Check sheet for the modelled part. Datum: model origin and axes. Units: mm. A direction names the side the tool comes from. Coordinates: 2 decimals unless noted, no trailing zeros. Loops run counter-clockwise (first coordinate to the right, second up) from the corner with the lowest first, then second, coordinate; pieces in that order, holes last. Notation, with made-up numbers: M -0.5,-37.75 L 49.5,-37.75 A19 cw 49.5,-29.75 Z; hole C -23.75,60 d5. An arc over 180 degrees is marked long. Write each question's results on one line, items separated by ' | '. Start each with the question number.
from build123d import *

# Parameters (mm, degrees)
BOSS_EXTRU_2_DEPTH = 2.4
CHANFREIN3_SIZE    = 1.4
CHANFREIN4_SIZE    = 1.4


with BuildPart() as part:
    # Esquisse2 → Boss.-Extru.2 (new body)
    with BuildSketch(Plane(origin=(0, 0, 0), x_dir=(1, 0, 0), z_dir=(0, 1, 0))):
        Polygon((-0.604426001, 3.317657231), (-4.604426001, 3.317657231), (-8.332361087, 1.867657231), (-8.332361087, -0.132342769), (-4.604426001, -1.582342769), (-0.604426001, -1.582342769), (3.123509084, -0.132342769), (3.123509084, 1.867657231), align=None)
        with BuildLine():
            Line((-0.204426001, 1.517657231), (-5.004426001, 1.517657231))
            ThreePointArc((-5.004426001, 1.517657231), (-5.654426001, 0.867657231), (-5.004426001, 0.217657231))
            Line((-5.004426001, 0.217657231), (-0.204426001, 0.217657231))
            ThreePointArc((-0.204426001, 0.217657231), (0.445573999, 0.867657231), (-0.204426001, 1.517657231))
        make_face(mode=Mode.SUBTRACT)
    extrude(amount=BOSS_EXTRU_2_DEPTH)

    # Chanfrein3
    chanfrein3_edges = [part.edges().sort_by_distance(p)[0] for p in [
        (-8.332361087, 2.4, -0.867657231),
    ]]
    chamfer(chanfrein3_edges, length=CHANFREIN3_SIZE)

    # Chanfrein4
    chanfrein4_edges = [part.edges().sort_by_distance(p)[0] for p in [
        (3.123509084, 2.4, -0.867657231),
    ]]
    chamfer(chanfrein4_edges, length=CHANFREIN4_SIZE)


solid = part.part
1) Section check D-D (x = -5.25). Enter the section's corners in (y, z).
2) Release check for a two-part mould opening along X. For faces 1 (the flat face through (-3, 0, 0)), 2 (the cylindrical face through (-5.654, 1.183, -0.882)), 3 (the flat face through (1.29, 1.18, -2.58)) record: +X half, -X half, draft (parallel to the pull), parting line (faces both ways), or undercut.
3) Set-up check for faces 4 (the flat face through (-6.442, 1.183, -2.603)), 5 (the cylindrical face through (0.445, 1.183, -0.853)): record each of +Z, -Z, +X, -X, +Y, -Y from which the full face is reachable in a straight line by a thin tool's end or side.
4) Section check C-C (y = 0.6). Enter the section's corners in (x, z).
5) Section check A-A (x = -3.5). Enter the section's corners in (y, z), then the cut area to 3 significant figures.
6) Thickness scan on probe 1 along Z at (x, y) = (-1.75, 1.7); probe 2 along X at (y, z) = (1.8, 0.05); probe 3 along X at (y, z) = (0.25, -1.3). Record the ranges inside material, lowest first.
7) Section check B-B (z = -1). Enter the section's corners in (x, y), then the cut area to 3 significant figures.
Return value:
1) outline: M 0,-3.07 L 2.4,-3.07 L 2.4,-1.47 L 0,-1.47 Z; M 0,-0.27 L 2.4,-0.27 L 2.4,1.33 L 0,1.33 Z
2) face 1: draft | face 2: undercut | face 3: +X half
3) face 4: -Z, -X, +Y, -Y | face 5: +Y, -Y
4) outline: M -8.33,-1.87 L -4.6,-3.32 L -0.6,-3.32 L 3.12,-1.87 L 3.12,0.13 L -0.6,1.58 L -4.6,1.58 L -8.33,0.13 Z; hole M -5,-1.52 L -0.2,-1.52 A0.65 ccw -0.2,-0.22 L -5,-0.22 A0.65 ccw Z
5) outline: M 0,-3.32 L 2.4,-3.32 L 2.4,-1.52 L 0,-1.52 Z; M 0,-0.22 L 2.4,-0.22 L 2.4,1.58 L 0,1.58 Z | area: 8.64 mm2
6) probe 1: z = -3.32 to -1.52, -0.22 to 1.58 | probe 2: x = -7.53 to 2.32 | probe 3: x = -8.33 to -5.49, 0.28 to 3.12
7) outline: M -8.33,0 L -5.64,0 L -5.64,2.4 L -6.93,2.4 L -8.33,1 Z; M 0.43,0 L 3.12,0 L 3.12,1 L 1.72,2.4 L 0.43,2.4 Z | area: 11.0 mm2
